from build123d import *

# Parameters (mm, degrees)
F0_W     = 99.2
F0_H     = 151.6
F0_W_2   = 92
F0_H_2   = 144.4
F0_W_3   = 85.6
F0_H_3   = 138
F1_DEPTH = 2.7
F2_DEPTH = 3.2
F3_SIZE  = 3.19999


# Not quite as in the source:
# - a fillet or chamfer is up to 0.001 mm smaller than in the source, because OpenCascade refuses the exact size


with BuildPart() as f1:
    # F0 (on Top) → F1 (new body)
    with BuildSketch(Plane.XY):
        Rectangle(F0_W, F0_H)
        Rectangle(F0_W_2, F0_H_2, mode=Mode.SUBTRACT)
        Rectangle(F0_W_2, F0_H_2)
        Rectangle(F0_W_3, F0_H_3, mode=Mode.SUBTRACT)
        Rectangle(F0_W_3, F0_H_3)
    extrude(amount=-F1_DEPTH)

    # F0 (on Top) → F2 (join)
    with BuildSketch(Plane.XY):
        Rectangle(F0_W_2, F0_H_2)
        Rectangle(F0_W_3, F0_H_3, mode=Mode.SUBTRACT)
        Rectangle(F0_W_3, F0_H_3)
    extrude(amount=F2_DEPTH)

    # F3 (size 3.2 in the source; OpenCascade refuses exactly that, so slightly less here)
    f3_edges = [f1.edges().sort_by_distance(p)[0] for p in [
        (0, -72.2, 3.2),
        (-46, 0, 3.2),
        (46, 0, 3.2),
        (0, 72.2, 3.2),
    ]]
    chamfer(f3_edges, length=F3_SIZE)


solid = f1.part
Geometry: final body of the model. Coordinates: model frame, mm. A direction names the side the tool comes from. Give positions to 0.01 mm unless a question says otherwise; leave off trailing zeros. Write each loop counter-clockwise with the first axis right and the second up, starting at its lowest first coordinate (ties: lowest second). Pieces come first, ordered by that corner, then holes. Notation, with made-up numbers: (-10.75, -18) -> (48.25, -18) arc R22 ccw to (48.25, 20) -> close; hole circle Ø1 at (32.25, 59.5). An arc over 180 degrees is marked (long way). Answer in a Markdown table with one row per item.
(1) Pin query (flat end, axial travel): pin 1 (1 mm diameter, centred on y = 57.5, z = 1.5, fed in from -X). Return the tip coordinate at first contact, or that it passes through.
Answers below:
| item | result |
|---|---|
| pin 1 | x = -45 |
(2) Section query C-C on z = 1. Return loops of the section in (x, y), then the cut area to 3 significant figures.
Answers below:
| item | result |
|---|---|
| outline | (-45, -71.2) -> (45, -71.2) -> (45, 71.2) -> (-45, 71.2) -> close |
| area | 12,800 mm^2 |
(3) Set-up query: faces 1 (the flat face through (44, -1, 2)), 2 (the flat face through (-48, 0, 0)). Return all of +Z, -Z, +X, -X, +Y, -Y with unobstructed straight access to the full face (end or side cutting, diameter ignored); none if empty.
Answers below:
| item | result |
|---|---|
| face 1 | +Z, +X, +Y, -Y |
| face 2 | +Z |
(4) Ray query, line 1 along Y through (x, z) = (11.5, 1.9); line 2 along X through (y, z) = (43, 0.55); line 3 along X through (y, z) = (28.5, 2.6). Return the intervals inside material, ascending. Write a range as [from, to].
Answers below:
| item | result |
|---|---|
| line 1 | [-70.3, 70.3] |
| line 2 | [-45.45, 45.45] |
| line 3 | [-43.4, 43.4] |
